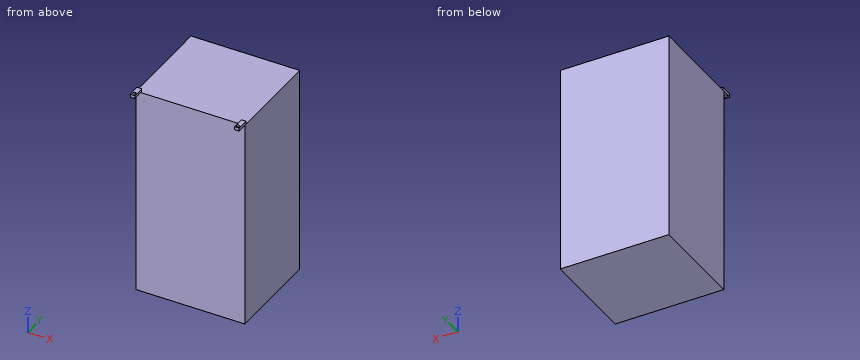
from build123d import *

# Parameters (mm, degrees)
F0_W     = 904.875
F0_H     = 1743.075
F1_DEPTH = 812.8
F2_W     = 38.1
F2_H     = 101.6
F2_R     = 12.7
F3_DEPTH = 25.4


with BuildPart() as f1:
    # F0 (on Front) → F1 (new body)
    with BuildSketch(Plane.XZ):
        with Locations((-1.664946, 168.443598)):
            Rectangle(F0_W, F0_H)
    extrude(amount=F1_DEPTH)

    # F2 (on face) → F3 (join)
    with BuildSketch(Plane.XY.offset(1039.981098)):
        with Locations((-433.464946, -850.9)):
            Rectangle(F2_W, F2_H)
        with Locations((-433.464946, -876.3)):
            Circle(F2_R, mode=Mode.SUBTRACT)
        with Locations((430.135054, -844.55)):
            Rectangle(F2_W, F2_H)
        with Locations((430.135054, -876.3)):
            Circle(F2_R, mode=Mode.SUBTRACT)
    extrude(amount=F3_DEPTH)


solid = f1.part
The listing builds one solid part. Answer for the finished solid, in the listing's coordinates (mm). Coordinates: 2 decimals unless noted, no trailing zeros. Order: outer loops, then holes, each group sorted by start corner. A loop starts at its lowest first (then second) coordinate and runs counter-clockwise, first axis right, second up.
Q1. A cutting plane is placed at B-B, the plane z = -261. Write down the section's boundary in (x, y), and give its area (3 significant figures).
Q2. Given P1, Ø4, axis at x = 272.5, y = -326, coming from the +Z side; P2, Ø12.5, axis at y = -854.5, z = 1050, coming from the -X side; P3, Ø23, axis at x = 430.14, y = -876.3, coming from the -Z side; P4, Ø7.5, axis at y = -826.5, z = 1058, coming from the +X side, each flat-ended and moving along its own axis, determine where each tip first touches the part or whether it passes through.
Q3. A cutting plane is placed at A-A, the plane x = -280. Write down the section's boundary in (y, z), and give its area (3 significant figures).
Q4. Consider line 1 (X direction, y = -876.3, z = 1054.5); line 2 (Z direction, x = -179, y = -758.5); line 3 (Y direction, x = -252, z = 59). Determine where each line is inside the solid, lowest interval first.
Answers follow:
1. outline: (-454.1, -812.8) - (450.77, -812.8) - (450.77, 0) - (-454.1, 0) - close
1. area: 735,000 mm2
2. P1: stops at z = 1039.98
2. P2: stops at x = -452.51
2. P3: passes through
2. P4: stops at x = 449.19
3. outline: (-812.8, -703.09) - (0, -703.09) - (0, 1039.98) - (-812.8, 1039.98) - close
3. area: 1,420,000 mm2
4. line 1: x = -452.51 to -446.16, -420.76 to -414.41, 411.09 to 417.44, 442.84 to 449.19
4. line 2: z = -703.09 to 1039.98
4. line 3: y = -812.8 to 0
